Source: CAD feature listing. Evaluate the final solid. Frame: model axes, mm. Face numbers are marked on the shaded views. A direction names the side the tool comes from. Give positions to 0.01 mm unless a question says otherwise; leave off trailing zeros. Answer in a Markdown table with one row per item.
```python
from build123d import *

# Parameters (mm, degrees)
SKETCH2_R               = 3.25
CUT_EXTRUDE1_DEPTH      = 9.138277453
CUT_EXTRUDE1_DEPTH_BACK = 9.799222547


with BuildPart() as part:
    # Sketch1 → Revolve1 (revolve)
    with BuildSketch(Plane(origin=(0, 0, 0), x_dir=(0, 0, -1), z_dir=(1, 0, 0))):
        Polygon((0.861722547, -29.175), (0.048922547, -29.175), (-0.967077453, -30.191), (-0.967077453, -61.484), (0.048922547, -62.5), (8.799222547, -62.5), (8.799222547, -73), (-3.126077453, -73), (-4.142077453, -71.984), (-4.142077453, -30.191), (-5.158077453, -29.175), (-7.122277453, -29.175), (-8.138277453, -28.159), (-8.138277453, -25), (-7.138277453, -25), (-7.138277453, -26), (-0.154277453, -26), (0.861722547, -27.016), align=None)
    revolve(axis=Axis((0, 0, 0), (0, 0, 1)))

    # Sketch2 → Cut-Extrude1 (cut, two sides)
    with BuildSketch(Plane.XY) as cut_extrude1_sk:
        with Locations((-58.52440797, -34.625043996)):
            Circle(SKETCH2_R)
        with Locations((-65.866609149, 16.899402332)):
            Circle(SKETCH2_R)
        with Locations((-34.625043996, 58.52440797)):
            Circle(SKETCH2_R)
        with Locations((16.899402332, 65.866609149)):
            Circle(SKETCH2_R)
        with Locations((58.52440797, 34.625043996)):
            Circle(SKETCH2_R)
        with Locations((65.866609149, -16.899402332)):
            Circle(SKETCH2_R)
        with Locations((34.625043996, -58.52440797)):
            Circle(SKETCH2_R)
        with Locations((-16.899402332, -65.866609149)):
            Circle(SKETCH2_R)
    extrude(amount=CUT_EXTRUDE1_DEPTH, mode=Mode.SUBTRACT)
    extrude(cut_extrude1_sk.sketch, amount=-CUT_EXTRUDE1_DEPTH_BACK, mode=Mode.SUBTRACT)


solid = part.part
```
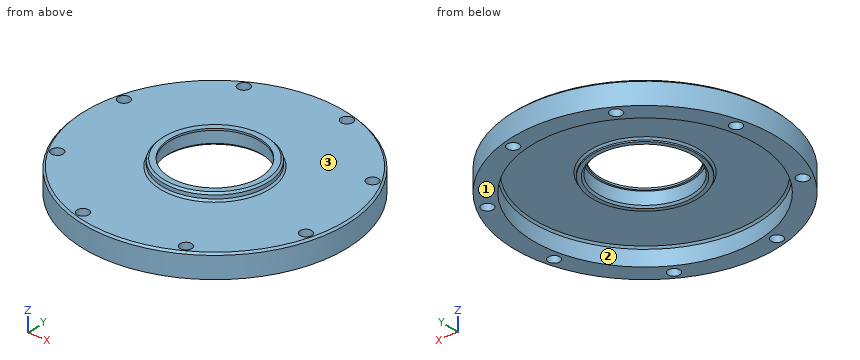
1) Set-up query: the marked faces 1, 2 and 3. Return all of +Z, -Z, +X, -X, +Y, -Y with unobstructed straight access to the full face (end or side cutting, diameter ignored); none if empty.
Reply:
| item | result |
|---|---|
| face 1 | -Z, +X, -X, +Y, -Y |
| face 2 | -Z |
| face 3 | +Z |
2) Section A-A, the plane z = -4.5. Count the separate pieces of the cut face and the enclosed holes in it, then the cut area to 3 significant figures.
Reply:
| item | result |
|---|---|
| separate pieces | 1 |
| enclosed holes | 9 |
| area | 4,200 mm² |
3) Material intervals for L1, parallel to X at y = 19.5, z = -6.75; L2, parallel to X at y = 36, z = -7.75; L3, parallel to X at y = 50.5, z = -4.25, sorted ascending.
Reply:
| item | result |
|---|---|
| L1 | x = -70.35 to -67.82, -63.92 to -59.38, 59.38 to 70.35 |
| L2 | x = -63.51 to -51.09, 51.09 to 55.58, 61.47 to 63.51 |
| L3 | x = -52.71 to -36.82, 36.82 to 52.71 |
4) Pin query (flat end, axial travel): pin 1 Ø5 at (x, y) = (-43, -53.5) entering from +Z; pin 2 Ø4 at (x, y) = (-46, -5.5) entering from -Z; pin 3 Ø1.5 at (x, z) = (29.5, -0.5) entering from -Y. Return the tip coordinate at first contact, or that it passes through.
Reply:
| item | result |
|---|---|
| pin 1 | stops at z = 4.14 |
| pin 2 | stops at z = 0.97 |
| pin 3 | stops at y = -67.1 |
